Drawing for the job (mm, zero at the part's lowest x, y, z). A direction names the side the tool comes from. Round coordinates to 2 decimals unless told otherwise and drop trailing zeros. Write each loop counter-clockwise with the first axis right and the second up, starting at its lowest first coordinate (ties: lowest second). Pieces come first, ordered by that corner, then holes. Notation, with made-up numbers: M 65.5,21 L 78.5,21 A20 ccw 78.5,36 Z; hole C -29,86 d4. An arc over 180 degrees is marked long. Use a Markdown table: item, result.
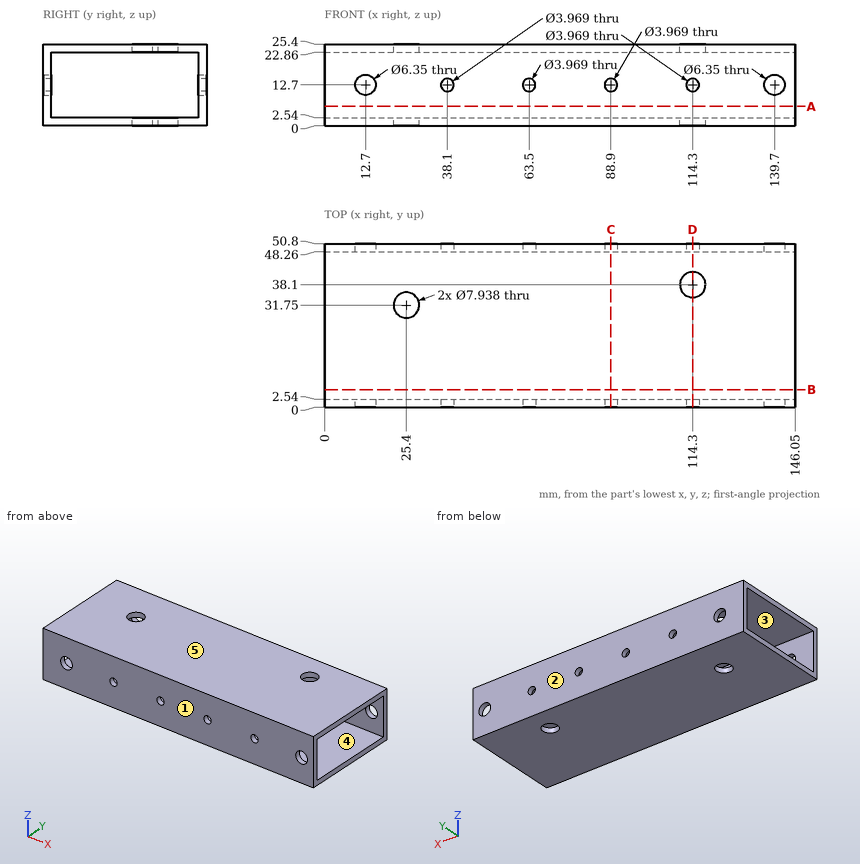
Q1. Cut at A-A on z = 6. Give the cut face in (x, y).
Response values:
| item | result |
|---|---|
| outline | M 0,0 L 146.05,0 L 146.05,2.54 L 0,2.54 Z; M 0,48.26 L 146.05,48.26 L 146.05,50.8 L 0,50.8 Z |
Q2. Drop flat-ended pins along their axis: P1, Ø5, axis at x = 139.7, z = 12.7, coming from the +Y side; P2, Ø1.5, axis at x = 20.5, z = 8.5, coming from the -Y side. Give the stop position or say it passes through.
Response values:
| item | result |
|---|---|
| P1 | passes through |
| P2 | stops at y = 0 |
Q3. Drill centre lines: L1, parallel to Z at x = 102.5, y = 29.5; L2, parallel to Y at x = 52.5, z = 15.25; L3, parallel to Y at x = 114.3, z = 0.5. Where is each one in solid material? Low to high.
Response values:
| item | result |
|---|---|
| L1 | z = 0 to 2.54, 22.86 to 25.4 |
| L2 | y = 0 to 2.54, 48.26 to 50.8 |
| L3 | y = 0 to 34.13, 42.07 to 50.8 |
Q4. Cut at D-D on x = 114.3. Give the cut face in (y, z) (1 decimal), and give its area (3 significant figures).
Response values:
| item | result |
|---|---|
| outline | M 0,0 L 34.1,0 L 34.1,2.5 L 2.5,2.5 L 2.5,10.7 L 0,10.7 Z; M 0,14.7 L 2.5,14.7 L 2.5,22.9 L 34.1,22.9 L 34.1,25.4 L 0,25.4 Z; M 42.1,0 L 50.8,0 L 50.8,10.7 L 48.3,10.7 L 48.3,2.5 L 42.1,2.5 Z; M 42.1,22.9 L 48.3,22.9 L 48.3,14.7 L 50.8,14.7 L 50.8,25.4 L 42.1,25.4 Z |
| area | 301 mm2 |
Q5. Two-plate mould, pull along Y, no slides. Class the marked faces 1, 2 and 3: +Y half, -Y half, draft (parallel to the pull), parting line (faces both ways), or undercut.
Response values:
| item | result |
|---|---|
| face 1 | -Y half |
| face 2 | +Y half |
| face 3 | undercut |
Q6. Which spindle directions (+Z, -Z, +X, -X, +Y, -Y) get a long thin tool onto all of the face, cutting with end or side? Do the marked faces 4 and 5. Say none if no direction does.
Response values:
| item | result |
|---|---|
| face 4 | +X, -X |
| face 5 | +Z, +X, -X, +Y, -Y |
Q7. Cut at C-C on x = 88.9. Give the cut face in (y, z) (1 decimal), and give its area (3 significant figures).
Response values:
| item | result |
|---|---|
| outline | M 0,0 L 50.8,0 L 50.8,10.7 L 48.3,10.7 L 48.3,2.5 L 2.5,2.5 L 2.5,10.7 L 0,10.7 Z; M 0,14.7 L 2.5,14.7 L 2.5,22.9 L 48.3,22.9 L 48.3,14.7 L 50.8,14.7 L 50.8,25.4 L 0,25.4 Z |
| area | 341 mm2 |
Q8. Cut at B-B on y = 5.5. Give the cut face in (x, z).
Response values:
| item | result |
|---|---|
| outline | M 0,0 L 146.05,0 L 146.05,2.54 L 0,2.54 Z; M 0,22.86 L 146.05,22.86 L 146.05,25.4 L 0,25.4 Z |
